Design review of the part built by this model. Coordinates are the model's own, in mm. A direction names the side the tool comes from. Round coordinates to 2 decimals unless told otherwise and drop trailing zeros. Loops run counter-clockwise (first coordinate to the right, second up) from the corner with the lowest first, then second, coordinate; pieces in that order, holes last. Notation, with made-up numbers: (26, 47.25) -> (68, 47.25) arc R22 ccw to (68, 59.25) -> close; hole circle Ø10 at (-11.5, 57). An arc over 180 degrees is marked (long way). Answer as CSV lines item,"result". Start each with the question number.
```python
from build123d import *

# Parameters (mm, degrees)
SKETCH6_W           = 100
SKETCH6_H           = 155
BOSS_EXTRUDE5_DEPTH = 55
FILLET2_R           = 5
SHELL3_START        = -45
SHELL3_OUTLINE_W    = 145
SHELL3_OUTLINE_H    = 50
SHELL3_DEPTH        = 90
BOSS_EXTRUDE6_DEPTH = 45
SKETCH8_R           = 2.1
CUT_EXTRUDE1_DEPTH  = 6.5
SKETCH9_R           = 2.5
SKETCH9_R_2         = 3
SKETCH9_R_3         = 7
CUT_EXTRUDE2_DEPTH  = 108.383657975
CUT_EXTRUDE3_REACH  = 173.901
CUT_EXTRUDE4_START  = -3
CUT_EXTRUDE4_DEPTH  = 3
BOSS_EXTRUDE7_DEPTH = 3


# Read off the part's stored shape, not the designer's step: Shell3
with BuildPart() as part:
    # Sketch6 → Boss-Extrude5 (new body)
    with BuildSketch(Plane.XY):
        Rectangle(SKETCH6_W, SKETCH6_H)
    extrude(amount=BOSS_EXTRUDE5_DEPTH)

    # Fillet2
    fillet2_edges = [part.edges().sort_by_distance(p)[0] for p in [
        (-50, 0, 55),
        (0, -77.5, 55),
        (50, 0, 55),
        (0, -77.5, 0),
        (-50, 0, 0),
        (0, 77.5, 0),
        (50, 0, 0),
        (50, -77.5, 27.5),
        (-50, -77.5, 27.5),
        (-50, 77.5, 27.5),
        (50, 77.5, 27.5),
        (0, 77.5, 55),
    ]]
    fillet(fillet2_edges, radius=FILLET2_R)

    # Shell3 outline → Shell3 (cut)
    with BuildSketch(Plane.YZ.offset(SHELL3_START)):
        with Locations((0, 25)):
            Rectangle(SHELL3_OUTLINE_W, SHELL3_OUTLINE_H)
    extrude(amount=SHELL3_DEPTH, mode=Mode.SUBTRACT)

    # Sketch7 → Boss-Extrude6 (add)
    with BuildSketch(Plane(origin=(0, 0, 50), x_dir=(-1, 0, 0), z_dir=(0, 0, -1))):
        with BuildLine():
            Line((-45, 72.5), (-37, 72.5))
            Line((-37, 72.5), (-37, 71.5))
            ThreePointArc((-37, 71.5), (-39.050252532, 66.550252532), (-44, 64.5))
            Line((-44, 64.5), (-45, 64.5))
            Line((-45, 64.5), (-45, 72.5))
        make_face()
        with BuildLine():
            Line((45, 72.5), (37, 72.5))
            Line((37, 72.5), (37, 71.5))
            ThreePointArc((37, 71.5), (39.050252532, 66.550252532), (44, 64.5))
            Line((44, 64.5), (45, 64.5))
            Line((45, 64.5), (45, 72.5))
        make_face()
        with BuildLine():
            Line((-45, -64.5), (-44, -64.5))
            ThreePointArc((-44, -64.5), (-39.050252532, -66.550252532), (-37, -71.5))
            Line((-37, -71.5), (-37, -72.5))
            Line((-37, -72.5), (-45, -72.5))
            Line((-45, -72.5), (-45, -64.5))
        make_face()
        with BuildLine():
            Line((45, -72.5), (45, -64.5))
            Line((45, -64.5), (44, -64.5))
            ThreePointArc((44, -64.5), (39.050252532, -66.550252532), (37, -71.5))
            Line((37, -71.5), (37, -72.5))
            Line((37, -72.5), (45, -72.5))
        make_face()
    extrude(amount=BOSS_EXTRUDE6_DEPTH)

    # Sketch8 → Cut-Extrude1 (cut)
    with BuildSketch(Plane(origin=(0, 0, 5), x_dir=(-1, 0, 0), z_dir=(0, 0, -1))):
        with Locations((-42, 69.5)):
            Circle(SKETCH8_R)
        with Locations((42, 69.5)):
            Circle(SKETCH8_R)
        with Locations((42, -69.5)):
            Circle(SKETCH8_R)
        with Locations((-42, -69.5)):
            Circle(SKETCH8_R)
    extrude(amount=-CUT_EXTRUDE1_DEPTH, mode=Mode.SUBTRACT)

    # Sketch9 → Cut-Extrude2 (cut, through all)
    with BuildSketch(Plane.XY.offset(55)):
        with Locations((0, 42.5)):
            Circle(SKETCH9_R)
        with Locations((0, 7.5)):
            Circle(SKETCH9_R_2)
        with Locations((0, -27.5)):
            Circle(SKETCH9_R_3)
    extrude(amount=-CUT_EXTRUDE2_DEPTH, mode=Mode.SUBTRACT)

    # Sketch10 → Cut-Extrude3 (cut, up to next)
    with BuildSketch(Plane.XZ.offset(77.5), mode=Mode.PRIVATE) as cut_extrude3_sk1:
        with BuildLine():
            Line((-3.5, 50), (3.5, 50))
            ThreePointArc((3.5, 50), (4.914213562, 49.414213562), (5.5, 48))
            Line((5.5, 48), (5.5, 47.8))
            ThreePointArc((5.5, 47.8), (4.914213562, 46.385786438), (3.5, 45.8))
            Line((3.5, 45.8), (-3.5, 45.8))
            ThreePointArc((-3.5, 45.8), (-4.914213562, 46.385786438), (-5.5, 47.8))
            Line((-5.5, 47.8), (-5.5, 48))
            ThreePointArc((-5.5, 48), (-4.914213562, 49.414213562), (-3.5, 50))
        make_face()
    cut_extrude3_tool1 = extrude(cut_extrude3_sk1.sketch, amount=-CUT_EXTRUDE3_REACH, mode=Mode.PRIVATE) & part.part
    add(cut_extrude3_tool1.solids().sort_by_distance((0, -77.5, 47.9))[0], mode=Mode.SUBTRACT)

    # Sketch13 → Cut-Extrude4 (cut)
    with BuildSketch(Plane(origin=(0, -72.5, 0), x_dir=(1, 0, 0), z_dir=(0, 1, 0)).offset(CUT_EXTRUDE4_START)):
        with BuildLine():
            Line((5.5, -47.8), (5.5, -48))
            ThreePointArc((5.5, -48), (5.457812626, -48.408619287), (5.333030278, -48.8))
            Line((5.333030278, -48.8), (10.333030278, -48.8))
            Line((10.333030278, -48.8), (10.333030278, -50))
            Line((10.333030278, -50), (3.5, -50))
            Line((3.5, -50), (-3.5, -50))
            Line((-3.5, -50), (-10.333030278, -50))
            Line((-10.333030278, -50), (-10.333030278, -48.8))
            Line((-10.333030278, -48.8), (-5.333030278, -48.8))
            ThreePointArc((-5.333030278, -48.8), (-5.457812626, -48.408619287), (-5.5, -48))
            Line((-5.5, -48), (-5.5, -47.8))
            ThreePointArc((-5.5, -47.8), (-4.914213562, -46.385786438), (-3.5, -45.8))
            Line((-3.5, -45.8), (3.5, -45.8))
            ThreePointArc((3.5, -45.8), (4.914213562, -46.385786438), (5.5, -47.8))
        make_face()
    extrude(amount=CUT_EXTRUDE4_DEPTH, mode=Mode.SUBTRACT)

    # Sketch14 → Boss-Extrude7 (add)
    with BuildSketch(Plane(origin=(0, 0, 50), x_dir=(-1, 0, 0), z_dir=(0, 0, -1))):
        with BuildLine():
            Line((-7.5, -46.6), (7.5, -46.5))
            Line((7.5, -46.5), (7.5, -46.6))
            ThreePointArc((7.5, -46.6), (6.943502884, -47.943502884), (5.6, -48.5))
            Line((5.6, -48.5), (-5.6, -48.5))
            ThreePointArc((-5.6, -48.5), (-6.943502884, -47.943502884), (-7.5, -46.6))
        make_face()
    extrude(amount=BOSS_EXTRUDE7_DEPTH)


solid = part.part
```
Q1. For pin 1 Ø2 at (x, y) = (-24.5, 17) entering from -Z; pin 2 Ø2.5 at (x, y) = (-9, -74.5) entering from +Z; pin 3 Ø1.3 at (x, y) = (-43, -69) entering from -Z; pin 4 Ø5.5 at (x, y) = (0, 7.5) entering from +Z (3 decimals), all flat-tipped, find the tip position at first contact; note any pin that passes through.
Q2. Machinability: for faces 1 (the flat face through (-8, -74, 48.8)), 2 (the cylindrical face through (0.63, -76.07, 1.5)), 3 (the flat face through (-42, 70, 11.5)), which of the approach directions +Z, -Z, +X, -X, +Y, -Y give a long, thin tool a straight path to every point of the face, cutting with its end or side? Answer none if there is none.
Q3. Add section C-C, the plane z = 28. Give the boundary of the cut face in (x, y).
Q4. Add section A-A, the plane y = 42.5. Give the boundary of the cut face in (x, z), and give its area (3 significant figures).
Q5. Add section B-B, the plane x = 0. Give the boundary of the cut face in (y, z), and give its area (3 significant figures).
Q6. Mouldability with a two-part tool opening along Y and no side actions: class faces 4 (the flat face through (-40, -68, 5)), 5 (the cylindrical face through (-49, 1, 53)), 6 (the cylindrical face through (-48.57, 76, 27.82)) as pulls with the +Y half, pulls with the -Y half, needs draft (parallel to the pull), parting line crosses it, or undercut.
Q7. Add section D-D, the plane y = -43.5. Give the boundary of the cut face in (x, z).
Q8. To check wall thickness, follow probe 1 along Y at (x, z) = (-18, 33.5); probe 2 along X at (y, z) = (56.5, 5); probe 3 along Y at (x, z) = (0, 53.6). State the ranges of each line that lie inside material, in increasing order. Write a range as from..to.
Worked answers:
1,pin 1,"stops at z = 50"
1,pin 2,"stops at z = 54.94"
1,pin 3,"stops at z = 11.5"
1,pin 4,"passes through"
2,face 1,"none"
2,face 2,"-Z, +X, -X, -Y"
2,face 3,"-Z"
3,outline,"(-50, -72.5) arc R5 ccw to (-45, -77.5) -> (45, -77.5) arc R5 ccw to (50, -72.5) -> (50, 72.5) arc R5 ccw to (45, 77.5) -> (-45, 77.5) arc R5 ccw to (-50, 72.5) -> close; hole (-45, -64.5) -> (-44, -64.5) arc R7 cw to (-37, -71.5) -> (-37, -72.5) -> (37, -72.5) -> (37, -71.5) arc R7 cw to (44, -64.5) -> (45, -64.5) -> (45, 64.5) -> (44, 64.5) arc R7 cw to (37, 71.5) -> (37, 72.5) -> (-37, 72.5) -> (-37, 71.5) arc R7 cw to (-44, 64.5) -> (-45, 64.5) -> close"
4,outline,"(-50, 5) arc R5 ccw to (-45, 0) -> (-45, 50) -> (-2.5, 50) -> (-2.5, 55) -> (-45, 55) arc R5 ccw to (-50, 50) -> close; (2.5, 50) -> (45, 50) -> (45, 0) arc R5 ccw to (50, 5) -> (50, 50) arc R5 ccw to (45, 55) -> (2.5, 55) -> close"
4,area,"954 mm^2"
5,outline,"(-77.5, 5) arc R5 ccw to (-72.5, 0) -> (-72.5, 45.8) -> (-77.5, 45.8) -> close; (-77.5, 50) -> (-48.5, 50) -> (-48.5, 47) -> (-46.55, 47) -> (-46.55, 50) -> (-34.5, 50) -> (-34.5, 55) -> (-72.5, 55) arc R5 ccw to start; (-20.5, 50) -> (4.5, 50) -> (4.5, 55) -> (-20.5, 55) -> close; (10.5, 50) -> (40, 50) -> (40, 55) -> (10.5, 55) -> close; (45, 50) -> (72.5, 50) -> (72.5, 0) arc R5 ccw to (77.5, 5) -> (77.5, 50) arc R5 ccw to (72.5, 55) -> (45, 55) -> close"
5,area,"1,110 mm^2"
6,face 4,"undercut"
6,face 5,"needs draft"
6,face 6,"pulls with the +Y half"
7,outline,"(-50, 5) arc R5 ccw to (-45, 0) -> (-45, 50) -> (45, 50) -> (45, 0) arc R5 ccw to (50, 5) -> (50, 50) arc R5 ccw to (45, 55) -> (-45, 55) arc R5 ccw to (-50, 50) -> close"
8,probe 1,"y = -77.5..-72.5, 72.5..77.5"
8,probe 2,"x = -50..-45, 45..50"
8,probe 3,"y = -75.97..-34.5, -20.5..4.5, 10.5..40, 45..75.97"
